Check sheet for the modelled part. Datum: model origin and axes. Units: mm. Face numbers are marked on the shaded views. A direction names the side the tool comes from. Give positions to 0.01 mm unless a question says otherwise; leave off trailing zeros. Write each loop counter-clockwise with the first axis right and the second up, starting at its lowest first coordinate (ties: lowest second). Pieces come first, ordered by that corner, then holes. Notation, with made-up numbers: (-35, -32.75) -> (24, -32.75) arc R24 cw to (24, 4.25) -> close; hole circle Ø5 at (85, 38.25). An arc over 180 degrees is marked (long way). Return JSON: item names as keys, results as strings.
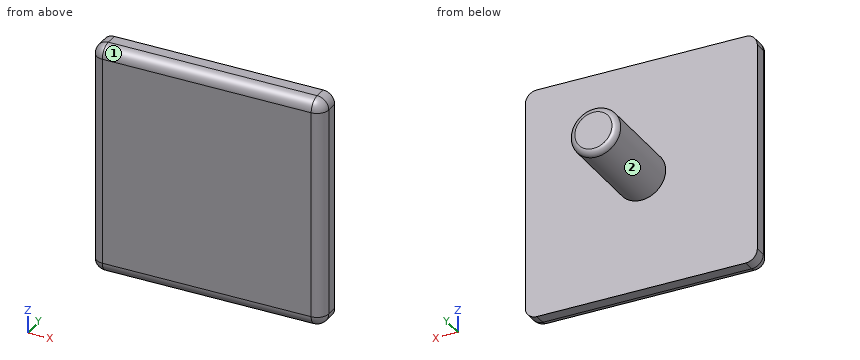
from build123d import *

# Parameters (mm, degrees)
SKETCH1_R           = 2.1
BOSS_EXTRUDE1_DEPTH = 8
SKETCH2_W           = 20
SKETCH2_H           = 20
BOSS_EXTRUDE2_DEPTH = 2
FILLET1_R           = 1
FILLET2_R           = 0.5
FILLET3_R           = 1


with BuildPart() as part:
    # Sketch1 → Boss-Extrude1 (new body)
    with BuildSketch(Plane(origin=(0, 0, 0), x_dir=(1, 0, 0), z_dir=(0, 1, 0))):
        with Locations(Location((10, 10, 0), (0, 0, 270))):
            Circle(SKETCH1_R)
    extrude(amount=BOSS_EXTRUDE1_DEPTH)

    # Sketch2 → Boss-Extrude2 (add)
    with BuildSketch(Plane.XZ):
        with Locations((10, -10)):
            Rectangle(SKETCH2_W, SKETCH2_H)
    extrude(amount=BOSS_EXTRUDE2_DEPTH)

    # Fillet1
    fillet1_edges = [part.edges().sort_by_distance(p)[0] for p in [
        (0, -2, -10),
        (10, -2, -20),
        (20, -2, -10),
        (10, -2, 0),
    ]]
    fillet(fillet1_edges, radius=FILLET1_R)

    # Fillet2
    fillet2_edges = [part.edges().sort_by_distance(p)[0] for p in [
        (10, 8, -12.1),
    ]]
    fillet(fillet2_edges, radius=FILLET2_R)

    # Fillet3
    # the kernel refuses this fillet: 1 mm, written as the material it takes off along each edge
    with BuildSketch(Plane(origin=(19, -1, -19), x_dir=(0, 0, -1), z_dir=(1, 0, 0))) as fillet3_piece_1_section:
        Polygon((0, 0), (FILLET3_R, 0), (FILLET3_R, -FILLET3_R), (0, -FILLET3_R), align=None)
    fillet3_piece_1 = extrude(amount=FILLET3_R, mode=Mode.PRIVATE)
    fillet3_piece_1 = fillet3_piece_1 - Plane(origin=(19, -1, -19), x_dir=(0, 0.7071067811865475, 0.7071067811865475), z_dir=(1, 0, 0)) * Sphere(FILLET3_R, mode=Mode.PRIVATE)
    add(fillet3_piece_1, mode=Mode.SUBTRACT)
    with BuildSketch(Plane(origin=(1, -1, -19), x_dir=(0, 0, -1), z_dir=(-1, 0, 0))) as fillet3_piece_2_section:
        Polygon((0, 0), (FILLET3_R, 0), (FILLET3_R, FILLET3_R), (0, FILLET3_R), align=None)
    fillet3_piece_2 = extrude(amount=FILLET3_R, mode=Mode.PRIVATE)
    fillet3_piece_2 = fillet3_piece_2 - Plane(origin=(1, -1, -19), x_dir=(0, 0.7071067811865475, 0.7071067811865475), z_dir=(-1, 0, 0)) * Sphere(FILLET3_R, mode=Mode.PRIVATE)
    add(fillet3_piece_2, mode=Mode.SUBTRACT)
    with BuildSketch(Plane(origin=(19, -1, -1), x_dir=(1, 0, 0), z_dir=(0, 0, 1))) as fillet3_piece_3_section:
        Polygon((0, 0), (FILLET3_R, 0), (FILLET3_R, -FILLET3_R), (0, -FILLET3_R), align=None)
    fillet3_piece_3 = extrude(amount=FILLET3_R, mode=Mode.PRIVATE)
    fillet3_piece_3 = fillet3_piece_3 - Plane(origin=(19, -1, -1), x_dir=(-0.7071067811865475, 0.7071067811865475, 0), z_dir=(0, 0, 1)) * Sphere(FILLET3_R, mode=Mode.PRIVATE)
    add(fillet3_piece_3, mode=Mode.SUBTRACT)
    with BuildSketch(Plane(origin=(1, -1, -1), x_dir=(-1, 0, 0), z_dir=(0, 0, 1))) as fillet3_piece_4_section:
        Polygon((0, 0), (FILLET3_R, 0), (FILLET3_R, FILLET3_R), (0, FILLET3_R), align=None)
    fillet3_piece_4 = extrude(amount=FILLET3_R, mode=Mode.PRIVATE)
    fillet3_piece_4 = fillet3_piece_4 - Plane(origin=(1, -1, -1), x_dir=(0.7071067811865475, 0.7071067811865475, 0), z_dir=(0, 0, 1)) * Sphere(FILLET3_R, mode=Mode.PRIVATE)
    add(fillet3_piece_4, mode=Mode.SUBTRACT)
    with BuildSketch(Plane(origin=(0, 2.5, 0), x_dir=(1, 0, 0), z_dir=(0, -1, 0)), Plane(origin=(0, 2.5, -20), x_dir=(0, 0, 1), z_dir=(0, -1, 0))) as fillet3_piece_5:
        with BuildLine():
            CenterArc((FILLET3_R, -FILLET3_R), FILLET3_R, 90, 90)
            Line((0, -FILLET3_R), (0, 0))
            Line((0, 0), (FILLET3_R, 0))
        make_face()
    extrude(amount=3.5, mode=Mode.SUBTRACT)
    with BuildSketch(Plane(origin=(20, 2.5, 0), x_dir=(-1, 0, 0), z_dir=(0, -1, 0)), Plane(origin=(20, 2.5, -20), x_dir=(0, 0, 1), z_dir=(0, -1, 0))) as fillet3_piece_6:
        with BuildLine():
            CenterArc((FILLET3_R, FILLET3_R), FILLET3_R, 180, 90)
            Line((0, FILLET3_R), (0, 0))
            Line((0, 0), (FILLET3_R, 0))
        make_face()
    extrude(amount=3.5, mode=Mode.SUBTRACT)


solid = part.part
(1) Cross-section at A-A on z = -4.5. Enter the section's corners in (x, y), then the cut area to 3 significant figures.
Reply:
{"outline": "(0, -1) arc R1 ccw to (1, -2) -> (19, -2) arc R1 ccw to (20, -1) -> (20, 0) -> (0, 0) -> close", "area": "39.6 mm^2"}
(2) Cross-section at C-C on y = 1.5. Enter the section's corners in (x, z).
Reply:
{"outline": "circle Ø4.2 at (10, -10)"}
(3) Thickness scan on L1, parallel to Y at x = 19, z = -10; L2, parallel to Z at x = 10.75, y = 2.5; L3, parallel to Z at x = 19.25, y = -1. Record the ranges inside material, lowest first.
Reply:
{"L1": "-2 to 0", "L2": "-11.96 to -8.04", "L3": "-19.97 to -0.03"}
(4) Depth check by flat-ended pin: pin 1 Ø2 at (x, y) = (12, 5.5) entering from -Z; pin 2 Ø3 at (y, z) = (5.5, -11) entering from +X; pin 3 Ø1 at (x, y) = (10.5, 5.5) entering from +Z. Enter the tip coordinate at first touch or a pass-through.
Reply:
{"pin 1": "z = -11.85", "pin 2": "x = 12.1", "pin 3": "z = -7.9"}
(5) Cross-section at B-B on x = 5.25. Enter the section's corners in (y, z), then the cut area to 3 significant figures.
Reply:
{"outline": "(-2, -19) arc R1 ccw to (-1, -20) -> (0, -20) -> (0, 0) -> (-1, 0) arc R1 ccw to (-2, -1) -> close", "area": "39.6 mm^2"}
(6) Set-up check for the marked faces 1 and 2: record each of +Z, -Z, +X, -X, +Y, -Y from which the full face is reachable in a straight line by a thin tool's end or side.
Reply:
{"face 1": "+Z, +X, -X, -Y", "face 2": "+Y"}
(7) Cross-section at D-D on z = -10. Enter the section's corners in (x, y), then the cut area to 3 significant figures.
Reply:
{"outline": "(0, -1) arc R1 ccw to (1, -2) -> (19, -2) arc R1 ccw to (20, -1) -> (20, 0) -> (12.1, 0) -> (12.1, 7.5) arc R0.5 ccw to (11.6, 8) -> (8.4, 8) arc R0.5 ccw to (7.9, 7.5) -> (7.9, 0) -> (0, 0) -> close", "area": "73.1 mm^2"}
